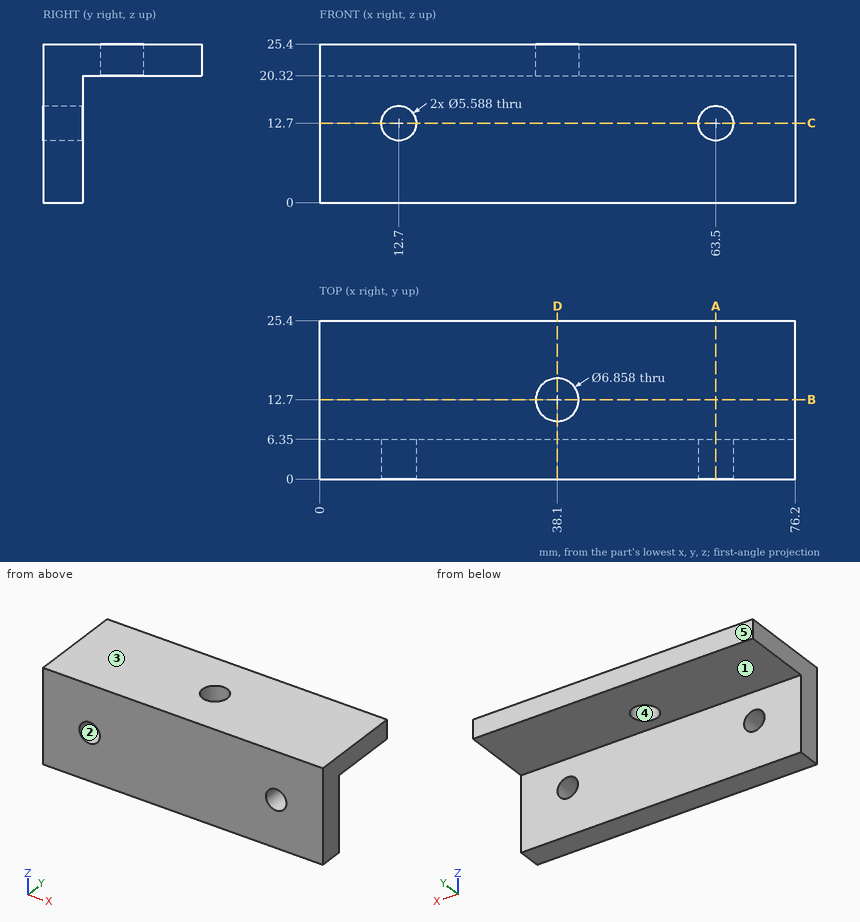
Job drawing, mm, ordinate dimensions from the low corner. One solid piece. A direction names the side the tool comes from. Coordinates: 2 decimals unless noted, no trailing zeros. Loops run counter-clockwise (first coordinate to the right, second up) from the corner with the lowest first, then second, coordinate; pieces in that order, holes last. Notation, with made-up numbers: (66, -13) - (125, -13) arc R14 ccw to (125, -6) - close; hole circle Ø4 at (-36, 68.5). An arc over 180 degrees is marked (long way). Write item = value, one per line. Start each with the question number.
Q1. Which spindle directions (+Z, -Z, +X, -X, +Y, -Y) get a long thin tool onto all of the face, cutting with end or side? Do the marked faces 1 and 2. Say none if no direction does.
Q2. Cut at D-D, the plane x = 38.1. List the corners of the cut face in (y, z).
Q3. Drill centre lines: L1, parallel to X at y = 3.25, z = 12.7; L2, parallel to Y at x = 17, z = 20; L3, parallel to Z at x = 51, y = 19.75. Where is each one in solid material? Low to high.
Q4. Pull direction Y, two halves, no side cores. Call the marked faces 3, 4 and 5: pulls with the +Y half, pulls with the -Y half, needs draft (parallel to the pull), parting line crosses it, or undercut.
Q5. Cut at C-C, the plane z = 12.7. List the corners of the cut face in (x, y).
Q6. Cut at B-B, the plane y = 12.7. List the corners of the cut face in (x, z).
Q7. Cut at A-A, the plane x = 63.5. List the corners of the cut face in (y, z), then the cut area to 3 significant figures.
Q8. Flat gauge pins, fed straight in: pin 1 Ø12 at (y, z) = (9, 7) entering from +X; pin 2 Ø6.5 at (x, z) = (63.5, 12.7) entering from +Y; pin 3 Ø3 at (x, y) = (62, 18.5) entering from -Z. Where does each tip first touch, or does it go through?
Computed:
q1.face_1 = -Z, +X, -X, +Y
q1.face_2 = +Y, -Y
q2.outline = (0, 0) - (6.35, 0) - (6.35, 20.32) - (9.27, 20.32) - (9.27, 25.4) - (0, 25.4) - close; (16.13, 20.32) - (25.4, 20.32) - (25.4, 25.4) - (16.13, 25.4) - close
q3.L1 = 0 to 9.91, 15.49 to 60.71, 66.29 to 76.2
q3.L2 = 0 to 6.35
q3.L3 = 20.32 to 25.4
q4.face_3 = needs draft
q4.face_4 = undercut
q4.face_5 = pulls with the +Y half
q5.outline = (0, 0) - (9.91, 0) - (9.91, 6.35) - (0, 6.35) - close; (15.49, 0) - (60.71, 0) - (60.71, 6.35) - (15.49, 6.35) - close; (66.29, 0) - (76.2, 0) - (76.2, 6.35) - (66.29, 6.35) - close
q6.outline = (0, 20.32) - (34.67, 20.32) - (34.67, 25.4) - (0, 25.4) - close; (41.53, 20.32) - (76.2, 20.32) - (76.2, 25.4) - (41.53, 25.4) - close
q7.outline = (0, 0) - (6.35, 0) - (6.35, 9.91) - (0, 9.91) - close; (0, 15.49) - (6.35, 15.49) - (6.35, 20.32) - (25.4, 20.32) - (25.4, 25.4) - (0, 25.4) - close
q7.area = 223 mm²
q8.pin_1 = 76.2
q8.pin_2 = 6.35
q8.pin_3 = 20.32
